Build history of the part. All positions in model axes, mm. Give positions to 0.01 mm unless a question says otherwise; leave off trailing zeros. Write each loop counter-clockwise with the first axis right and the second up, starting at its lowest first coordinate (ties: lowest second). Pieces come first, ordered by that corner, then holes.
from build123d import *

# Parameters (mm, degrees)
SKETCH1_W           = 25.4
SKETCH1_H           = 107.95
SKETCH1_R           = 3.175
BOSS_EXTRUDE1_DEPTH = 3.175


with BuildPart() as part:
    # Sketch1 → Boss-Extrude1 (new body)
    with BuildSketch(Plane.XZ.offset(3.175)):
        with Locations((-0.642134808, -2.283393272)):
            Rectangle(SKETCH1_W, SKETCH1_H)
        with Locations((-0.642134808, -49.908393272)):
            Circle(SKETCH1_R, mode=Mode.SUBTRACT)
        with Locations((-0.642134808, 45.341606728)):
            Circle(SKETCH1_R, mode=Mode.SUBTRACT)
    extrude(amount=-BOSS_EXTRUDE1_DEPTH)


solid = part.part
(1) Drop flat-ended pins along their axis: pin 1 (4 mm diameter, centred on x = -0.64, z = -49.91, fed in from +Y); pin 2 (10 mm diameter, centred on x = -10.5, z = 35, fed in from +Y). Give the stop position or say it passes through.
(2) Mould opens along X. For faces 1 (the face through (12.058, -2, -3)), 2 (the face through (-1, -2, 51.692)), 3 (the face through (-1.33, -1.61, 42.24)) say: +X half, -X half, draft (parallel to the pull), parting line (faces both ways), or undercut.
(3) Saw through at B-B, the plane z = -48.5. List the corners of the cut face in (x, y) (3 decimals), plus the area to 3 significant figures.
(4) Saw through at C-C, the plane y = -1.65. List the corners of the cut face in (x, z) (3 decimals), plus the area to 3 significant figures.
(5) Probe line 1 (Z direction, x = -2.75, y = -1.35); line 2 (Z direction, x = -3, y = -2.15); line 3 (X direction, y = -2.05, z = 47.5). List the from-to ranges inside material, lowest first.
(6) Saw through at A-A, the plane x = 0.25. List the corners of the cut face in (y, z) (3 decimals).
Computed values:
1. pin 1: passes through
1. pin 2: stops at y = 0
2. face 1: +X half
2. face 2: draft
2. face 3: undercut
3. outline: (-13.342, -3.175) - (-3.488, -3.175) - (-3.488, 0) - (-13.342, 0) - close; (2.203, -3.175) - (12.058, -3.175) - (12.058, 0) - (2.203, 0) - close
3. area: 62.6 mm2
4. outline: (-13.342, -56.258) - (12.058, -56.258) - (12.058, 51.692) - (-13.342, 51.692) - close; hole circle Ø6.35 at (-0.642, -49.908); hole circle Ø6.35 at (-0.642, 45.342)
4. area: 2,680 mm2
5. line 1: z = -56.26 to -52.28, -47.53 to 42.97, 47.72 to 51.69
5. line 2: z = -56.26 to -52.03, -47.78 to 43.22, 47.47 to 51.69
5. line 3: x = -13.34 to -2.97, 1.69 to 12.06
6. outline: (-3.175, -56.258) - (0, -56.258) - (0, -52.955) - (-3.175, -52.955) - close; (-3.175, -46.861) - (0, -46.861) - (0, 42.295) - (-3.175, 42.295) - close; (-3.175, 48.389) - (0, 48.389) - (0, 51.692) - (-3.175, 51.692) - close
